```python
from build123d import *

# Parameters (mm, degrees)
SKETCH_1_R               = 18
EXTRUDE_1_DEPTH          = 40
CUT_EXTRUDE_2_DEPTH      = 88.891979156
CUT_EXTRUDE_2_DEPTH_BACK = 88.891979156
SKETCH_2_R               = 9
SKETCH_3_R               = 10.1
CUT_EXTRUDE_3_DEPTH      = 15
CUT_EXTRUDE_START        = -15
SKETCH_4_R               = 10.1
CUT_EXTRUDE_4_DEPTH      = 15
CUT_EXTRUDE_5_DEPTH      = 88.891979202
CUT_EXTRUDE_5_DEPTH_BACK = 88.891979202
SKETCH_5_R               = 9
SKETCH_6_R               = 10.1
CUT_EXTRUDE_6_DEPTH      = 15
CUT_EXTRUDE_START_2      = -8
SKETCH_7_R               = 10.1
CUT_EXTRUDE_7_DEPTH      = 8
EXTRUDE_2_DEPTH          = 2
FILLET_1_R               = 10
EXTRUDE_START            = 20
SKETCH_10_R              = 20.1
EXTRUDE_3_DEPTH          = 20
FILLET_2_R               = 4


with BuildPart() as part:
    # Эскиз1 → Бобышка-Вытянуть1 (new body)
    with BuildSketch(Plane(origin=(0, 0, 0), x_dir=(1, 0, 0), z_dir=(0, 1, 0))):
        with BuildLine():
            Line((19, 35), (-19, 35))
            ThreePointArc((-19, 35), (-30.313708499, 30.313708499), (-35, 19))
            Line((-35, 19), (-35, -19))
            ThreePointArc((-35, -19), (-30.313708499, -30.313708499), (-19, -35))
            Line((-19, -35), (19, -35))
            ThreePointArc((19, -35), (30.313708499, -30.313708499), (35, -19))
            Line((35, -19), (35, 19))
            ThreePointArc((35, 19), (30.313708499, 30.313708499), (19, 35))
        make_face()
        with Locations(Location((0, 0, 0), (0, 0, 270))):
            Circle(SKETCH_1_R, mode=Mode.SUBTRACT)
    extrude(amount=EXTRUDE_1_DEPTH)

    # Эскиз2 → Вырез-Вытянуть2 (cut, two sides: drawn at the far end of the back side and taken through both)
    with BuildSketch(Plane.ZY.offset(35).offset(-CUT_EXTRUDE_2_DEPTH_BACK)):
        with Locations((0, 20)):
            Circle(SKETCH_2_R)
    extrude(amount=CUT_EXTRUDE_2_DEPTH + CUT_EXTRUDE_2_DEPTH_BACK, mode=Mode.SUBTRACT)

    # Эскиз3 → Вырез-Вытянуть3 (cut)
    with BuildSketch(Plane.ZY.offset(35)):
        with Locations((0, 20)):
            Circle(SKETCH_3_R)
    extrude(amount=-CUT_EXTRUDE_3_DEPTH, mode=Mode.SUBTRACT)

    # Эскиз4 → Вырез-Вытянуть4 (cut)
    with BuildSketch(Plane(origin=(35, 0, 0), x_dir=(0, 0, -1), z_dir=(1, 0, 0)).offset(CUT_EXTRUDE_START)):
        with Locations(Location((0, 20, 0), (0, 0, 180))):
            Circle(SKETCH_4_R)
    extrude(amount=CUT_EXTRUDE_4_DEPTH, mode=Mode.SUBTRACT)

    # Эскиз5 → Вырез-Вытянуть5 (cut, two sides: drawn at the far end of the back side and taken through both)
    with BuildSketch(Plane.XY.offset(35).offset(-CUT_EXTRUDE_5_DEPTH_BACK)):
        with Locations((0, 20)):
            Circle(SKETCH_5_R)
    extrude(amount=CUT_EXTRUDE_5_DEPTH + CUT_EXTRUDE_5_DEPTH_BACK, mode=Mode.SUBTRACT)

    # Эскиз6 → Вырез-Вытянуть6 (cut)
    with BuildSketch(Plane.XY.offset(35)):
        with Locations((0, 20)):
            Circle(SKETCH_6_R)
    extrude(amount=-CUT_EXTRUDE_6_DEPTH, mode=Mode.SUBTRACT)

    # Эскиз7 → Вырез-Вытянуть7 (cut)
    with BuildSketch(Plane(origin=(0, 0, -35), x_dir=(-1, 0, 0), z_dir=(0, 0, -1)).offset(CUT_EXTRUDE_START_2)):
        with Locations(Location((0, 20, 0), (0, 0, 180))):
            Circle(SKETCH_7_R)
    extrude(amount=CUT_EXTRUDE_7_DEPTH, mode=Mode.SUBTRACT)

    # Эскиз9 → Бобышка-Вытянуть2 (add)
    with BuildSketch(Plane(origin=(0, 40, 0), x_dir=(1, 0, 0), z_dir=(0, 1, 0))):
        with BuildLine():
            Line((35, -19), (35, 19))
            ThreePointArc((35, 19), (30.313708499, 30.313708499), (19, 35))
            Line((19, 35), (-19, 35))
            ThreePointArc((-19, 35), (-30.313708499, 30.313708499), (-35, 19))
            Line((-35, 19), (-35, -19))
            ThreePointArc((-35, -19), (-30.313708499, -30.313708499), (-19, -35))
            Line((-19, -35), (19, -35))
            ThreePointArc((19, -35), (30.313708499, -30.313708499), (35, -19))
        make_face()
    extrude(amount=EXTRUDE_2_DEPTH)

    # Скругление1
    fillet_1_edges = [part.edges().sort_by_distance(p)[0] for p in [
        (30.313708499, 42, 30.313708499),
        (35, 42, 0),
        (30.313708499, 42, -30.313708499),
        (0, 42, -35),
        (-30.313708499, 42, -30.313708499),
        (-35, 42, 0),
        (-30.313708499, 42, 30.313708499),
        (0, 42, 35),
    ]]
    fillet(fillet_1_edges, radius=FILLET_1_R)

    # Эскиз10 → Бобышка-Вытянуть3 (add)
    with BuildSketch(Plane.XZ.offset(EXTRUDE_START)):
        with BuildLine():
            Line((19, 35), (-19, 35))
            ThreePointArc((-19, 35), (-30.313708499, 30.313708499), (-35, 19))
            Line((-35, 19), (-35, -19))
            ThreePointArc((-35, -19), (-30.313708499, -30.313708499), (-19, -35))
            Line((-19, -35), (19, -35))
            ThreePointArc((19, -35), (30.313708499, -30.313708499), (35, -19))
            Line((35, -19), (35, 19))
            ThreePointArc((35, 19), (30.313708499, 30.313708499), (19, 35))
        make_face()
        with Locations(Location((0, 0, 0), (0, 0, 270))):
            Circle(SKETCH_10_R, mode=Mode.SUBTRACT)
    extrude(amount=-EXTRUDE_3_DEPTH)

    # Скругление2
    fillet_2_edges = [part.edges().sort_by_distance(p)[0] for p in [
        (30.313708499, -20, 30.313708499),
        (0, -20, 35),
        (-30.313708499, -20, 30.313708499),
        (-35, -20, 0),
        (-30.313708499, -20, -30.313708499),
        (0, -20, -35),
        (30.313708499, -20, -30.313708499),
        (35, -20, 0),
    ]]
    fillet(fillet_2_edges, radius=FILLET_2_R)


solid = part.part
```
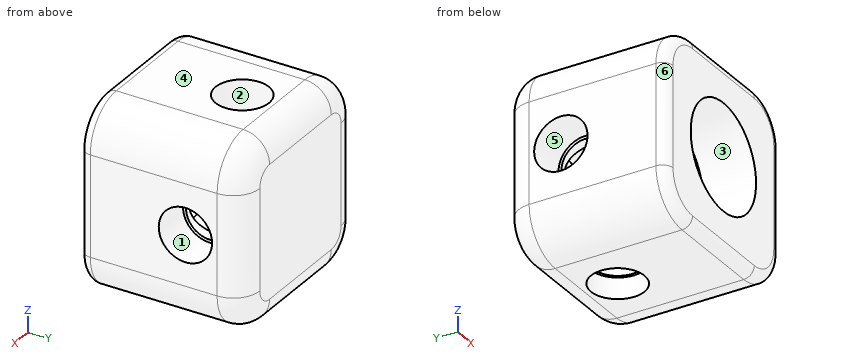
Source: CAD feature listing. Evaluate the final solid. Frame: model axes, mm. Face numbers are marked on the shaded views. A direction names the side the tool comes from. Give positions to 0.01 mm unless a question says otherwise; leave off trailing zeros. Order: outer loops, then holes, each group sorted by start corner. A loop starts at its lowest first (then second) coordinate and runs counter-clockwise, first axis right, second up.
(1) Section query D-D (x = 12). Return the cut outline in (y, z).
(2) Contact query for flat-ended pins moving along their axis: P1, Ø8, axis at x = -27, y = -5, coming from the +Z side; P2, Ø10, axis at y = 18.5, z = -4.5, coming from the +X side. Output: stop coordinate, or through.
(3) Pull-direction query (Y, two-part tool) for the marked faces 4, 5 and 6; classes: +Y half, -Y half, draft (parallel to the pull), parting line (faces both ways), or undercut.
(4) Section query C-C (y = 2.5). Return the cut outline in (x, z).
(5) Access query for the marked faces 1, 2 and 3. Directions: +Z, -Z, +X, -X, +Y, -Y. A direction counts if a zero-diameter tool reaches every point of the face in a straight line with its end or side. Return the directions, or none.
(6) Material intervals for line 1 along Z through (x, y) = (18.05, 20); line 2 along Y through (x, z) = (0, -31); line 3 along Y through (x, z) = (23.25, 0), sorted ascending.
(7) Section query A-A (x = 0). State how many separate pieces and enclosed holes the cut face has, plus the area to 3 significant figures.
Outcome:
1. outline: (-20, -31) arc R4 ccw to (-16, -35) - (32, -35) arc R10 ccw to (42, -25) - (42, 25) arc R10 ccw to (32, 35) - (-16, 35) arc R4 ccw to (-20, 31) - (-20, 16.12) - (0, 16.12) - (0, 13.42) - (40, 13.42) - (40, -13.42) - (0, -13.42) - (0, -16.12) - (-20, -16.12) - close
2. P1: stops at z = 34.49
2. P2: stops at x = 20
3. face 4: draft
3. face 5: undercut
3. face 6: -Y half
4. outline: (-35, -19) arc R16 ccw to (-19, -35) - (19, -35) arc R16 ccw to (35, -19) - (35, 19) arc R16 ccw to (19, 35) - (-19, 35) arc R16 ccw to (-35, 19) - close; hole circle Ø36 at (0, 0)
5. face 1: +X
5. face 2: +Z
5. face 3: -Y
6. line 1: z = -35 to -9, 9 to 35
6. line 2: y = -20 to 9.9, 30.1 to 40
6. line 3: y = -20 to 9.9, 30.1 to 42
7. separate pieces: 3
7. enclosed holes: 0
7. area: 1,380 mm2
